```python
from build123d import *

# Parameters (mm, degrees)
SKETCH1_R           = 1.85
BOSS_EXTRUDE1_DEPTH = 3.1
SKETCH2_R           = 1.5
BOSS_EXTRUDE2_DEPTH = 1
SKETCH3_R           = 1.1
BOSS_EXTRUDE3_DEPTH = 2


with BuildPart() as part:
    # Sketch1 → Boss-Extrude1 (new body)
    with BuildSketch(Plane(origin=(0, 0, 0), x_dir=(1, 0, 0), z_dir=(0, 1, 0))):
        with Locations(Location((0, 0, 0), (0, 0, 90))):
            Circle(SKETCH1_R)
    extrude(amount=BOSS_EXTRUDE1_DEPTH)

    # Sketch2 → Boss-Extrude2 (add)
    with BuildSketch(Plane(origin=(0, 3.1, 0), x_dir=(1, 0, 0), z_dir=(0, 1, 0))):
        with Locations(Location((0, 0, 0), (0, 0, 270))):
            Circle(SKETCH2_R)
    extrude(amount=BOSS_EXTRUDE2_DEPTH)

    # Sketch3 → Boss-Extrude3 (add)
    with BuildSketch(Plane(origin=(0, 4.1, 0), x_dir=(1, 0, 0), z_dir=(0, 1, 0))):
        with Locations(Location((0, 0, 0), (0, 0, 270))):
            Circle(SKETCH3_R)
    extrude(amount=BOSS_EXTRUDE3_DEPTH)

    # Loft1: read off the stored shape, not the designer's step
    # Loft1: loft between two sections, ruled curve by curve
    loft1_from = [
        Edge.make_bspline([(0, 6.1, 1.85), (3.7, 6.1, 1.85), (3.7, 6.1, -1.85), (0, 6.1, -1.85), (-3.7, 6.1, -1.85), (-3.7, 6.1, 1.85), (0, 6.1, 1.85)], [0, 0, 0, 0, 0.5, 0.5, 0.5, 1, 1, 1, 1], 3, [1, 0.333333333, 0.333333333, 1, 0.333333333, 0.333333333, 1]),
    ]
    loft1_to = [
        Edge.make_bspline([(0.620465421, 8.6, 0.968257539), (2.556980499, 8.6, -0.272673303), (1.316049657, 8.6, -2.209188381), (-0.620465421, 8.6, -0.968257539), (-2.556980499, 8.6, 0.272673303), (-1.316049657, 8.6, 2.209188381), (0.620465421, 8.6, 0.968257539)], [0, 0, 0, 0, 0.5, 0.5, 0.5, 1, 1, 1, 1], 3, [1, 0.333333333, 0.333333333, 1, 0.333333333, 0.333333333, 1]),
    ]
    loft1 = Solid(Shell([*[Face.make_surface_from_curves(loft1_from[k], loft1_to[k]) for k in range(1)], Face(Wire(loft1_from)), Face(Wire(loft1_to))]))
    add(loft1)


solid = part.part
```
The listing builds one solid part. Answer for the finished solid, in the listing's coordinates (mm). A direction names the side the tool comes from. Give positions to 0.01 mm unless a question says otherwise; leave off trailing zeros. Order: outer loops, then holes, each group sorted by start corner. A loop starts at its lowest first (then second) coordinate and runs counter-clockwise, first axis right, second up. Notation, with made-up numbers: (-20, -11.5) -> (-14, -11.5) arc R12 ccw to (-14, 7.5) -> close; hole circle Ø10 at (-26.75, 62.5). An arc over 180 degrees is marked (long way). Write each question's results on one line, items separated by ' | '.
Q1. Each of these flat-tipped pins is pushed along its axis until it touches: P1, Ø1.5, axis at y = 7, z = -1, coming from the -X side; P2, Ø1.5, axis at y = 3.5, z = -0.5, coming from the -X side. Where does it stop, or does it pass through?
Checked values:
P1: stops at x = -1.66 | P2: stops at x = -1.85
Q2. The part is cut by section A-A, the plane y = 0.5. Give the vertices of the cut face in (x, z), and give its area (3 significant figures).
Checked values:
outline: circle Ø3.7 at (0, 0) | area: 10.8 mm^2
Q3. Determine the mould class of faces 1 (the face through (0, 0, 0)), 2 (the face through (0.45, 3.59, 1.43)), 3 (the face through (1.806, 1.528, 0.401)), 4 (the face through (1.09, 5.09, -0.14)) for opening direction Y: pulls with the +Y half, pulls with the -Y half, needs draft (parallel to the pull), parting line crosses it, or undercut.
Checked values:
face 1: pulls with the -Y half | face 2: undercut | face 3: needs draft | face 4: undercut
Q4. Straight lines are drawn through the part: probe 1 along Y at (x, z) = (1, 1.15); probe 2 along Z at (x, y) = (0.1, 1); probe 3 along X at (y, z) = (5.5, -0.3). For each, find the intervals that lie inside material, in ascending order. Write a range as from..to.
Checked values:
probe 1: y = 0..3.1, 6.1..7.08 | probe 2: z = -1.85..1.85 | probe 3: x = -1.06..1.06
Q5. Which of the six approach directions +Z, -Z, +X, -X, +Y, -Y give full straight-line access (tool end or side, diameter ignored) to faces 5 (the face through (1, 6.1, 1)), 6 (the face through (0, 8.6, 0))?
Checked values:
face 5: none | face 6: +Z, -Z, +X, -X, +Y
Q6. The part is cut by section B-B, the plane y = 4.75. Give the vertices of the cut face in (x, z), and give its area (3 significant figures).
Checked values:
outline: circle Ø2.2 at (0, 0) | area: 3.80 mm^2
